from build123d import *

# Parameters (mm, degrees)
CYLINDER009_R     = 1.8
CYLINDER009_DEPTH = 20
ARRAY005_X_COUNT  = 2
ARRAY005_X_PITCH  = 68
ARRAY005_Y_COUNT  = 2
ARRAY005_Y_PITCH  = 58
CYLINDER005_R     = 1.2
CYLINDER005_DEPTH = 10
ARRAY003_X_COUNT  = 2
ARRAY003_X_PITCH  = 65.5
ARRAY003_Y_COUNT  = 2
ARRAY003_Y_PITCH  = 45.5
BOX006_W          = 74
BOX006_H          = 64
BOX006_DEPTH      = 3


with BuildPart() as wall_box_hole_stand_array001:
    # Cylinder009 → Cylinder009 (new body)
    with BuildSketch(Plane(origin=(3, 3, 0), x_dir=(1, 0, 0), z_dir=(0, 0, 1))):
        Circle(CYLINDER009_R)
    extrude(amount=CYLINDER009_DEPTH)

    # Array005 X: wall box hole stand array001 ×2


with BuildPart() as wall_box_hole_stand_array001_1:
    add(wall_box_hole_stand_array001.part)
    with Locations(*[(i * ARRAY005_X_PITCH, 0, 0) for i in range(1, ARRAY005_X_COUNT)]):
        add(wall_box_hole_stand_array001.part)

    # Array005 Y: wall box hole stand array001 ×2


with BuildPart() as wall_box_hole_stand_array001_2:
    add(wall_box_hole_stand_array001_1.part)
    with Locations(*[(0, i * ARRAY005_Y_PITCH, 0) for i in range(1, ARRAY005_Y_COUNT)]):
        add(wall_box_hole_stand_array001_1.part)


with BuildPart() as bottom_plate_hole_fusion:
    # Cylinder005 → Cylinder005 (new body)
    with BuildSketch(Plane.XY):
        Circle(CYLINDER005_R)
    extrude(amount=CYLINDER005_DEPTH)

    # Array003 X: bottom plate hole fusion ×2


with BuildPart() as bottom_plate_hole_fusion_1:
    add(bottom_plate_hole_fusion.part)
    with Locations(*[(i * ARRAY003_X_PITCH, 0, 0) for i in range(1, ARRAY003_X_COUNT)]):
        add(bottom_plate_hole_fusion.part)

    # Array003 Y: bottom plate hole fusion ×2


with BuildPart() as bottom_plate_hole_fusion_2:
    add(bottom_plate_hole_fusion_1.part)
    with Locations(*[(0, i * ARRAY003_Y_PITCH, 0) for i in range(1, ARRAY003_Y_COUNT)]):
        add(bottom_plate_hole_fusion_1.part)


with BuildPart() as bottom_plate_hole_fusion_3:
    # Array003 placement: moved
    add(bottom_plate_hole_fusion_2.part.moved(Location((4.25, 9.25, -3))))

    # Fusion004: union wall box hole stand array001
    add(wall_box_hole_stand_array001_2.part)


with BuildPart() as bottom_plate_cut:
    # Box006 → Box006 (new body)
    with BuildSketch(Plane.XY):
        with Locations((37, 32)):
            Rectangle(BOX006_W, BOX006_H)
    extrude(amount=BOX006_DEPTH)

    # Cut003: cut bottom plate hole fusion
    add(bottom_plate_hole_fusion_3.part, mode=Mode.SUBTRACT)


solid = bottom_plate_cut.part
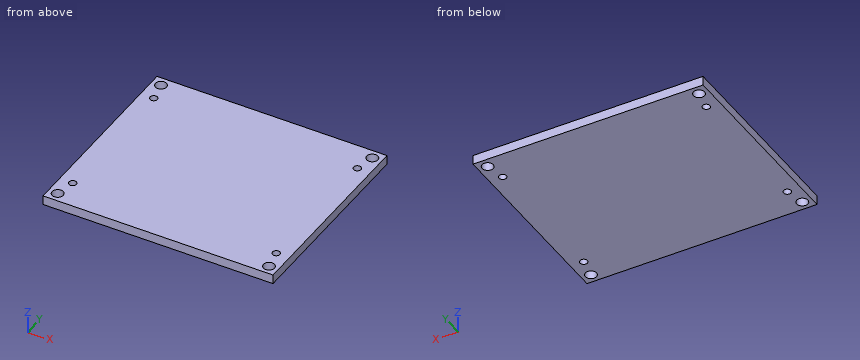
Design review of the part built by this model. Coordinates are the model's own, in mm. Give positions to 0.01 mm unless a question says otherwise; leave off trailing zeros. Order: outer loops, then holes, each group sorted by start corner. A loop starts at its lowest first (then second) coordinate and runs counter-clockwise, first axis right, second up.
1. For pin 1 Ø1.9 at (x, y) = (69.75, 9.25) entering from -Z, flat-tipped, find the tip position at first contact; note if it passes through.
Solution:
pin 1: passes through
2. Add section A-A, the plane y = 54.75. State the section outline as (x, z) points.
Solution:
outline: (0, 0) - (3.05, 0) - (3.05, 3) - (0, 3) - close; (5.45, 0) - (68.55, 0) - (68.55, 3) - (5.45, 3) - close; (70.95, 0) - (74, 0) - (74, 3) - (70.95, 3) - close
3. To check wall thickness, follow L1, parallel to X at y = 54.75, z = 2.2; L2, parallel to Y at x = 3, z = 1.65; L3, parallel to X at y = 3, z = 1.55. State the ranges of each line that lie inside material, in increasing order.
Solution:
L1: x = 0 to 3.05, 5.45 to 68.55, 70.95 to 74
L2: y = 0 to 1.2, 4.8 to 59.2, 62.8 to 64
L3: x = 0 to 1.2, 4.8 to 69.2, 72.8 to 74
